Design review of the part built by this model. Coordinates are the model's own, in mm. A direction names the side the tool comes from. Coordinates: 2 decimals unless noted, no trailing zeros. Loops run counter-clockwise (first coordinate to the right, second up) from the corner with the lowest first, then second, coordinate; pieces in that order, holes last. Notation, with made-up numbers: (13, 40) -> (47, 40) arc R19 cw to (47, 65) -> close; hole circle Ø10 at (-3.5, -24.5). An arc over 180 degrees is marked (long way). One line per item, written item: value. Start each with the question number.
1. Machinability: for faces 3 (the cylindrical face through (-24.1, -1.2, 1.5)), 4 (the cylindrical face through (-14.9, -1.8, 115.7)), which of the approach directions +Z, -Z, +X, -X, +Y, -Y give a long, thin tool a straight path to every point of the face, cutting with its end or side? Answer none if there is none.
2. Draft analysis for pull direction X (two halves, no side actions). For faces 1 (the cylindrical face through (10, 0, 116)), 2 (the flat face through (13, 0, 231.6)), state which applies: pulls with the +X half, pulls with the -X half, needs draft (parallel to the pull), parting line crosses it, or undercut.
3. Add section B-B on x = 22.5. Write out the cut boundary in (y, z), plus the area to 3 significant figures.
4. Add section A-A on y = 0. Write out the cut boundary in (x, z).
5. Insertion check: pin 1 (3 mm diameter, centred on x = 11.5, z = 194.5, fed in from +Y); pin 2 (4 mm diameter, centred on x = 20, y = -2, fed in from +Z); pin 3 (6 mm diameter, centred on y = 1.5, z = 187.5, fed in from -X). Each pin has a flat end and moves straight along its axis. Give the tip position at first contact, or say it passes through.
6. Add section C-C on z = 121.5. Write out the cut boundary in (x, y), plus the area to 3 significant figures.
7. For probe 1 along X at (y, z) = (0.25, 166); probe 2 along Y at (x, z) = (-22.5, 0.95); probe 3 along Z at (x, y) = (18.5, -6.5), list the stretches that pass through material, from the lowest coordinate up.
8. Add section D-D on x = -12.5. Write out the cut boundary in (y, z).
```python
from build123d import *

# Parameters (mm, degrees)
SKETCH1_W           = 55
SKETCH1_H           = 16
SKETCH1_R           = 2
BOSS_EXTRUDE1_DEPTH = 3
SKETCH3_R           = 3
BOSS_EXTRUDE2_DEPTH = 228.6


with BuildPart() as part:
    # Sketch1 → Boss-Extrude1 (new body)
    with BuildSketch(Plane.XY):
        Rectangle(SKETCH1_W, SKETCH1_H)
        with Locations((-22.5, 0)):
            Circle(SKETCH1_R, mode=Mode.SUBTRACT)
        with Locations((22.5, 0)):
            Circle(SKETCH1_R, mode=Mode.SUBTRACT)
    extrude(amount=BOSS_EXTRUDE1_DEPTH)

    # Sketch3 → Boss-Extrude2 (add)
    with BuildSketch(Plane.XY.offset(3)):
        with Locations((-12.5, 0)):
            Circle(SKETCH3_R)
        with Locations((13, 0)):
            Circle(SKETCH3_R)
    extrude(amount=BOSS_EXTRUDE2_DEPTH)


solid = part.part
```
Worked answers:
1. face 3: +Z, -Z
1. face 4: +Z
2. face 1: undercut
2. face 2: needs draft
3. outline: (-8, 0) -> (-2, 0) -> (-2, 3) -> (-8, 3) -> close; (2, 0) -> (8, 0) -> (8, 3) -> (2, 3) -> close
3. area: 36.0 mm²
4. outline: (-27.5, 0) -> (-24.5, 0) -> (-24.5, 3) -> (-27.5, 3) -> close; (-20.5, 0) -> (20.5, 0) -> (20.5, 3) -> (16, 3) -> (16, 231.6) -> (10, 231.6) -> (10, 3) -> (-9.5, 3) -> (-9.5, 231.6) -> (-15.5, 231.6) -> (-15.5, 3) -> (-20.5, 3) -> close; (24.5, 0) -> (27.5, 0) -> (27.5, 3) -> (24.5, 3) -> close
5. pin 1: stops at y = 3
5. pin 2: stops at z = 3
5. pin 3: stops at x = -15.5
6. outline: circle Ø6 at (-12.5, 0); circle Ø6 at (13, 0)
6. area: 56.5 mm²
7. probe 1: x = -15.49 to -9.51, 10.01 to 15.99
7. probe 2: y = -8 to -2, 2 to 8
7. probe 3: z = 0 to 3
8. outline: (-8, 0) -> (8, 0) -> (8, 3) -> (3, 3) -> (3, 231.6) -> (-3, 231.6) -> (-3, 3) -> (-8, 3) -> close
